Autodesk Inventor part; units mm, degrees
ref_plane "YZ Plane" through (0, 0, 0) normal (1, 0, 0) x (0, 1, 0)
ref_plane "XZ Plane" through (0, 0, 0) normal (0, 1, 0) x (-1, 0, 0)
ref_plane "XY Plane" through (0, 0, 0) normal (0, 0, 1) x (1, 0, 0)
sketch "スケッチ1" plane through (0, 0, 0) normal (0, 0, 1) x (1, 0, 0)
  circle A0 centre (0, 0) radius 1.65
  dimension "d0" = 3.3
extrude "押し出し1" add sketch "スケッチ1" along normal blind 30
sketch "スケッチ2" plane through (0, 0, 30) normal (0, 0, 1) x (1, 0, 0)
  circle A0 centre (0, 0) radius 4
  dimension "d3" = 8
extrude "押し出し2" add sketch "スケッチ2" against normal blind 2.3
chamfer "面取り1" distance 2.3 angle 45 1 edges at (-4, 0, 27.7)
thread "ねじ1"
properties part number "ネジ皿m4,30" material "鋼、高強度、低合金"
Here's how the part is built. I have some questions about the finished solid (model axes, mm). A direction names the side the tool comes from. Coordinates: 2 decimals unless noted, no trailing zeros. Order: outer loops, then holes, each group sorted by start corner. A loop starts at its lowest first (then second) coordinate and runs counter-clockwise, first axis right, second up.
1) I need wall thicknesses on line 1 (X direction, y = 0, z = 11.75); line 2 (Z direction, x = -2.5, y = -1); line 3 (X direction, y = 1.25, z = 25.5). Which ranges of each line are inside material? Lowest first, please.
2) Which directions (+Z, -Z, +X, -X, +Y, -Y) give clear straight access to the entire face, cutting with the end or side of a thin tool? Please do faces 1 (the face through (-1.216, -1.115, 13.656)), 2 (the face through (0, 0, 30)).
3) Will these pins go through, and if not, where does the flat tip stop? pin 1 (1 mm diameter, centred on x = 0, y = 1, fed in from -Z); pin 2 (1.5 mm diameter, centred on y = 1.5, z = 16, fed in from -X); pin 3 (1 mm diameter, centred on y = -0.5, z = 4, fed in from +X).
4) Imagine slicing it at C-C on z = 20. List the corners of the cut face in (x, y) for me, and give its area (3 significant figures).
Response values:
1. line 1: x = -1.65 to 1.65
1. line 2: z = 28.69 to 30
1. line 3: x = -1.08 to 1.08
2. face 1: -Z
2. face 2: +Z, +X, -X, +Y, -Y
3. pin 1: stops at z = 0
3. pin 2: stops at x = -1.47
3. pin 3: stops at x = 1.65
4. outline: circle Ø3.3 at (0, 0)
4. area: 8.55 mm2
